```python
from build123d import *

# Parameters (mm, degrees)
F0_W     = 190.5
F0_H     = 152.4
F0_W_2   = 168.91
F0_H_2   = 137.16
F1_DEPTH = 12.7
F3_R     = 5.08
F4_R     = 3.175
F5_R     = 1.27
F6_R     = 1.27
F7_START = -5.08
F2_W     = 69.85
F2_H     = 1.524
F7_DEPTH = 140.97
F8_DEPTH = 152.401


with BuildPart() as f1:
    # F0 (on Front) → F1 (new body)
    with BuildSketch(Plane.XZ):
        with Locations((95.25, 76.2)):
            Rectangle(F0_W, F0_H)
        with Locations((98.425, 76.2)):
            Rectangle(F0_W_2, F0_H_2, mode=Mode.SUBTRACT)
    extrude(amount=-F1_DEPTH)

    # F3
    f3_edges = [f1.edges().sort_by_distance(p)[0] for p in [
        (190.5, 6.35, 152.4),
    ]]
    fillet(f3_edges, radius=F3_R)

    # F4
    f4_edges = [f1.edges().sort_by_distance(p)[0] for p in [
        (190.5, 6.35, 0),
    ]]
    fillet(f4_edges, radius=F4_R)

    # F5
    f5_edges = [f1.edges().sort_by_distance(p)[0] for p in [
        (0, 0, 76.2),
        (0, 12.7, 76.2),
    ]]
    fillet(f5_edges, radius=F5_R)

    # F6
    f6_edges = [f1.edges().sort_by_distance(p)[0] for p in [
        (93.345, 0, 152.4),
        (1.27, 0, 76.2),
    ]]
    fillet(f6_edges, radius=F6_R)

    # F2 (on face) → F7 (cut)
    with BuildSketch(Plane.XY.offset(152.4).offset(F7_START)):
        with Locations((-34.925, 6.35)):
            Rectangle(F2_W, F2_H)
        with BuildLine():
            ThreePointArc((3.2677960807, 5.588), (3.175, 6.35), (3.2677960807, 7.112))
            Line((3.2677960807, 7.112), (0, 7.112))
            Line((0, 7.112), (0, 5.588))
            Line((0, 5.588), (3.2677960807, 5.588))
        make_face()
        with BuildLine():
            ThreePointArc((9.4322039193, 5.588), (9.5017155998, 5.9661852294), (9.525, 6.35))
            ThreePointArc((9.525, 6.35), (9.5017155998, 6.7338147706), (9.4322039193, 7.112))
            Line((9.4322039193, 7.112), (3.2677960807, 7.112))
            ThreePointArc((3.2677960807, 7.112), (3.175, 6.35), (3.2677960807, 5.588))
            Line((3.2677960807, 5.588), (9.4322039193, 5.588))
        make_face()
        with BuildLine():
            ThreePointArc((9.4322039193, 7.112), (9.5017155998, 6.7338147706), (9.525, 6.35))
            ThreePointArc((9.525, 6.35), (9.5017155998, 5.9661852294), (9.4322039193, 5.588))
            Line((9.4322039193, 5.588), (184.15, 5.588))
            Line((184.15, 5.588), (184.15, 7.112))
            Line((184.15, 7.112), (9.4322039193, 7.112))
        make_face()
    extrude(amount=-F7_DEPTH, mode=Mode.SUBTRACT)

    # F2 (on face) → F8 (cut, through all)
    with BuildSketch(Plane.XY.offset(152.4)):
        with BuildLine():
            ThreePointArc((9.4322039193, 5.588), (9.5017155998, 5.9661852294), (9.525, 6.35))
            ThreePointArc((9.525, 6.35), (9.5017155998, 6.7338147706), (9.4322039193, 7.112))
            Line((9.4322039193, 7.112), (3.2677960807, 7.112))
            ThreePointArc((3.2677960807, 7.112), (3.175, 6.35), (3.2677960807, 5.588))
            Line((3.2677960807, 5.588), (9.4322039193, 5.588))
        make_face()
        with BuildLine():
            ThreePointArc((3.2677960807, 5.588), (6.35, 3.175), (9.4322039193, 5.588))
            Line((9.4322039193, 5.588), (3.2677960807, 5.588))
        make_face()
        with BuildLine():
            Line((3.2677960807, 7.112), (9.4322039193, 7.112))
            ThreePointArc((9.4322039193, 7.112), (6.35, 9.525), (3.2677960807, 7.112))
        make_face()
    extrude(amount=-F8_DEPTH, mode=Mode.SUBTRACT)


solid = f1.part
```
Could you check a few things on this model? Use its own coordinates, in mm. A direction names the side the tool comes from. Give positions to 0.01 mm unless a question says otherwise; leave off trailing zeros. Write each loop counter-clockwise with the first axis right and the second up, starting at its lowest first coordinate (ties: lowest second). Pieces come first, ordered by that corner, then holes. Notation, with made-up numbers: (48, 82) - (69, 82) arc R8 ccw to (69, 95) - close; hole circle Ø9 at (67.25, -7). An arc over 180 degrees is marked (long way). One line per item, written item: value. Start each with the question number.
Item 1: I'm going to push a flat-ended pin straight in: pin 1 (1.7 mm diameter, centred on y = 6, z = 62.5, fed in from -X). Where does the tip first touch, or does it pass through?
Item 2: If we mould it in two halves opening along Z, with no side actions, what happens to faces 4 (the face through (93, 6, 0)), 5 (the face through (97, 3, 7.62)), 6 (the face through (92, 6, 152.4))? For each: +Z half, -Z half, draft (parallel to the pull), parting line (faces both ways), or undercut.
Item 3: Imagine slicing it at B-B, the plane x = 179.5. List the corners of the cut face in (y, z) for me, and give its area (3 significant figures).
Item 4: Please list where these lines run through material, in increasing order: line 1 (Z direction, x = 59, y = 8); line 2 (X direction, y = 10, z = 143); line 3 (X direction, y = 3.75, z = 25.5). Write a range as from..to.
Item 5: Which directions (+Z, -Z, +X, -X, +Y, -Y) give clear straight access to the entire face, cutting with the end or side of a thin tool? Please do faces 1 (the face through (58, 7.112, 145)), 2 (the face through (11, 0, 77)), 3 (the face through (97, 10, 144.78)).
Item 6: Imagine slicing it at A-A, the plane z = 58. List the corners of the cut face in (x, y) for me (3 decimals).
Geometry says:
1. pin 1: x = 0
2. face 4: -Z half
2. face 5: undercut
2. face 6: +Z half
3. outline: (0, 1.27) arc R1.27 ccw to (1.27, 0) - (11.43, 0) arc R1.27 ccw to (12.7, 1.27) - (12.7, 7.62) - (7.11, 7.62) - (7.11, 6.35) - (5.59, 6.35) - (5.59, 7.62) - (0, 7.62) - close; (0, 144.78) - (5.59, 144.78) - (5.59, 147.32) - (7.11, 147.32) - (7.11, 144.78) - (12.7, 144.78) - (12.7, 151.13) arc R1.27 ccw to (11.43, 152.4) - (1.27, 152.4) arc R1.27 ccw to (0, 151.13) - close
3. area: 186 mm^2
4. line 1: 0..7.62, 144.78..152.4
4. line 2: 0..13.97, 182.88..190.5
4. line 3: 0..4.53, 8.17..13.97, 182.88..190.5
5. face 1: -X
5. face 2: +Z, -Z, +X, -X, -Y
5. face 3: +Y, -Y
6. outline: (0, 1.27) arc R1.27 ccw to (1.27, 0) - (13.97, 0) - (13.97, 5.588) - (9.432, 5.588) arc R3.175 cw to (3.268, 5.588) - (0, 5.588) - close; (0, 7.112) - (3.268, 7.112) arc R3.175 cw to (9.432, 7.112) - (13.97, 7.112) - (13.97, 12.7) - (1.27, 12.7) arc R1.27 ccw to (0, 11.43) - close; (182.88, 0) - (189.23, 0) arc R1.27 ccw to (190.5, 1.27) - (190.5, 11.43) arc R1.27 ccw to (189.23, 12.7) - (182.88, 12.7) - (182.88, 7.112) - (184.15, 7.112) - (184.15, 5.588) - (182.88, 5.588) - close
